Geometry check sheet. Reference: the model listing, model coordinates, mm. A direction names the side the tool comes from. Give positions to 0.01 mm unless a question says otherwise; leave off trailing zeros. Write each loop counter-clockwise with the first axis right and the second up, starting at its lowest first coordinate (ties: lowest second). Pieces come first, ordered by that corner, then holes. Notation, with made-up numbers: (18, -24.5) - (65, -24.5) arc R29 cw to (65, 11.5) - close; hole circle Ø6 at (26.25, 44). An arc over 180 degrees is marked (long way). Write item = value, one per line. Start each with the question number.
(1) Depth check by flat-ended pin: pin 1 Ø0.5 at (x, y) = (9, 18) entering from +Z; pin 2 Ø8 at (x, y) = (-2.5, 9.5) entering from -Z; pin 3 Ø0.5 at (x, z) = (-13.5, -5.5) entering from -Y; pin 4 Ø3.5 at (x, z) = (-12, 1) entering from +Y. Enter the tip coordinate at first touch or a pass-through.
(2) Thickness scan on L1, parallel to X at y = 14.5, z = 6; L2, parallel to X at y = 14.25, z = 21; L3, parallel to Z at x = -5.5, y = 11.75. Record the ranges inside material, lowest first.
(3) Section check A-A, the plane y = 19.75. Enter the section's corners in (x, z), plus the area to 3 significant figures.
(4) Access from +Z, -Z, +X, -X, +Y, -Y to the whole of each face (thin tool, end or side, straight path). Record for faces 1 (the flat face through (13, 21, 18)), 2 (the flat face through (12, 19, 23)), 3 (the flat face through (13.5, 18, -18)), 4 (the cylindrical face through (-0.037, 13.325, -19.232)).
(5) Draft check along X on faces 5 (the cylindrical face through (0.19, 0.45, -19.57)), 6 (the flat face through (-13.75, 21.5, -7.6)), 7 (the cylindrical face through (-0.163, 7.526, -19.232)). Enter one of: pulls with the +X half, pulls with the -X half, needs draft (parallel to the pull), parting line crosses it, or undercut.
```python
from build123d import *

# Parameters (mm, degrees)
BOSS_EXTRUDE1_DEPTH      = 17.5
CUT_EXTRUDE1_DEPTH       = 14
CUT_EXTRUDE2_DEPTH       = 54.247065647
SKETCH4_W                = 26
SKETCH4_H                = 8
CUT_EXTRUDE3_DEPTH       = 1
BOSS_EXTRUDE3_DEPTH      = 7.5
BOSS_EXTRUDE3_DEPTH_BACK = 1
SKETCH6_W                = 5.4
SKETCH6_H                = 36
FILLET2_R                = 2
FILLET5_R                = 1.5
SKETCH13_W               = 15.2
SKETCH13_H               = 28
BOSS_EXTRUDE7_DEPTH      = 4
SKETCH15_R               = 1
CUT_EXTRUDE8_DEPTH       = 6
CHAMFER5_SIZE            = 6
SKETCH16_W               = 11
SKETCH16_H               = 5.5
BOSS_EXTRUDE8_DEPTH      = 2
SKETCH17_W               = 11
SKETCH17_H               = 5.5
BOSS_EXTRUDE9_DEPTH      = 2
BOSS_EXTRUDE14_START     = -2
BOSS_EXTRUDE14_DEPTH     = 0.5
CHAMFER6_SIZE            = 0.5
BOSS_EXTRUDE15_DEPTH     = 0.5
CHAMFER7_SIZE            = 0.5
CUT_EXTRUDE9_REACH       = 59.483
BOSS_EXTRUDE16_DEPTH     = 1
FILLET7_R                = 1
SKETCH27_W               = 11
SKETCH27_H               = 2
BOSS_EXTRUDE17_DEPTH     = 0.75
SKETCH27_3_W             = 11
SKETCH27_3_H             = 2.5
CUT_EXTRUDE10_DEPTH      = 0.3
SKETCH29_W               = 11
SKETCH29_H               = 2
BOSS_EXTRUDE18_DEPTH     = 0.75
SKETCH29_4_W             = 11
SKETCH29_4_H             = 2.5
CUT_EXTRUDE11_DEPTH      = 0.3
FILLET8_R                = 1


# Some blends are built 0.0001 mm under size
with BuildPart() as part:
    # Sketch1 → Boss-Extrude1 (new body)
    with BuildSketch(Plane(origin=(0, 0, 0), x_dir=(1, 0, 0), z_dir=(0, 1, 0))):
        Polygon((-15, 20), (15, 20), (15, -20), (15, -30), (-15, -30), (-15, -20), align=None)
    extrude(amount=BOSS_EXTRUDE1_DEPTH)

    # Sketch2 → Cut-Extrude1 (cut)
    with BuildSketch(Plane(origin=(0, 17.5, 0), x_dir=(1, 0, 0), z_dir=(0, 1, 0))):
        Polygon((-13, 18), (13, 18), (13, -18), (13, -28), (-13, -28), (-13, -18), align=None)
    extrude(amount=-CUT_EXTRUDE1_DEPTH, mode=Mode.SUBTRACT)

    # Sketch3 → Cut-Extrude2 (cut, through all)
    with BuildSketch(Plane.XY.offset(-18)):
        with BuildLine():
            ThreePointArc((2.74956137, 10.425664385), (-0.1, 13.325664385), (-2.94956137, 10.425664385))
            ThreePointArc((-2.94956137, 10.425664385), (-0.1, 7.525664385), (2.74956137, 10.425664385))
        make_face()
    extrude(amount=-CUT_EXTRUDE2_DEPTH, mode=Mode.SUBTRACT)

    # Sketch4 → Cut-Extrude3 (cut)
    with BuildSketch(Plane(origin=(0, 3.5, 0), x_dir=(1, 0, 0), z_dir=(0, 1, 0))):
        with Locations((0, 14)):
            Rectangle(SKETCH4_W, SKETCH4_H)
    extrude(amount=-CUT_EXTRUDE3_DEPTH, mode=Mode.SUBTRACT)

    # Sketch6 → Boss-Extrude3 (add, two sides: drawn at the far end of the back side and taken through both)
    with BuildSketch(Plane(origin=(0, 3.5, 0), x_dir=(1, 0, 0), z_dir=(0, 1, 0)).offset(-BOSS_EXTRUDE3_DEPTH_BACK)):
        with Locations((-10.3, 0)):
            Rectangle(SKETCH6_W, SKETCH6_H)
        with Locations((10.3, 0)):
            Rectangle(SKETCH6_W, SKETCH6_H)
    extrude(amount=BOSS_EXTRUDE3_DEPTH + BOSS_EXTRUDE3_DEPTH_BACK)

    # Fillet2
    fillet2_edges = [part.edges().sort_by_distance(p)[0] for p in [
        (-7.6, 11, 0),
        (7.6, 11, 0),
    ]]
    fillet(fillet2_edges, radius=FILLET2_R)

    # Fillet5
    fillet5_edges = [part.edges().sort_by_distance(p)[0] for p in [
        (15, 8.75, 30),
        (-15, 8.75, 30),
        (-15, 8.75, -20),
        (15, 8.75, -20),
        (0, 0, 30),
        (-15, 0, 5),
        (0, 0, -20),
        (15, 0, 5),
    ]]
    fillet(fillet5_edges, radius=FILLET5_R)

    # Sketch13 → Boss-Extrude7 (add)
    with BuildSketch(Plane(origin=(0, 3.5, 0), x_dir=(1, 0, 0), z_dir=(0, 1, 0))):
        with Locations((0, -4)):
            Rectangle(SKETCH13_W, SKETCH13_H)
    extrude(amount=BOSS_EXTRUDE7_DEPTH)

    # Sketch15 → Cut-Extrude8 (cut)
    with BuildSketch(Plane(origin=(0, 7.5, 0), x_dir=(1, 0, 0), z_dir=(0, 1, 0))):
        with Locations(Location((0, -8.82, 0), (0, 0, 270))):
            Circle(SKETCH15_R)
    extrude(amount=-CUT_EXTRUDE8_DEPTH, mode=Mode.SUBTRACT)

    # Chamfer5
    # the kernel refuses this chamfer: 6 mm, written as the material it takes off along each edge
    with BuildSketch(Plane(origin=(-7.6, 7.5, -10), x_dir=(0, -0.9996219169112968, -0.02749587661058649), z_dir=(1, 0, 0))) as chamfer5_piece_1_section:
        Polygon((CHAMFER5_SIZE * 0.999621916911, -CHAMFER5_SIZE * 0.0274958766106), (-CHAMFER5_SIZE * 0.0274958766106, -CHAMFER5_SIZE * 0.999621916911), (0, 0), align=None)
    chamfer5_piece_1 = extrude(amount=15.2, mode=Mode.PRIVATE)
    chamfer5_piece_1 = split(chamfer5_piece_1, bisect_by=Plane(origin=(0, 2.5, -7.952380952), z_dir=(0, 1, 0)), keep=Keep.TOP, mode=Mode.PRIVATE)
    add(chamfer5_piece_1, mode=Mode.SUBTRACT)

    # Sketch16 → Boss-Extrude8 (add)
    with BuildSketch(Plane(origin=(-13, 0, 0), x_dir=(0, 0, -1), z_dir=(1, 0, 0))):
        Polygon((2, 17.5), (2, 14.5), (2, 12), (13, 12), (13, 14.5), (13, 17.5), align=None)
        with Locations((7.5, 20.25)):
            Rectangle(SKETCH16_W, SKETCH16_H)
    extrude(amount=BOSS_EXTRUDE8_DEPTH)

    # Sketch17 → Boss-Extrude9 (add)
    with BuildSketch(Plane.ZY.offset(-13)):
        with Locations((17.5, 20.25)):
            Rectangle(SKETCH17_W, SKETCH17_H)
        Polygon((12, 17.5), (12, 14.5), (12, 12), (23, 12), (23, 14.5), (23, 17.5), align=None)
    extrude(amount=BOSS_EXTRUDE9_DEPTH)

    # Sketch3<4> → Boss-Extrude14 (add)
    with BuildSketch(Plane.XY.offset(-18).offset(BOSS_EXTRUDE14_START)):
        Polygon((-4.129390667, 8.806636123), (-1.769028262, 6.446273719), (1.569028262, 6.446273719), (3.929390667, 8.806636123), (3.929390667, 12.144692648), (1.569028262, 14.505055052), (-1.769028262, 14.505055052), (-4.129390667, 12.144692648), align=None)
        with BuildLine():
            ThreePointArc((-2.94956137, 10.425664385), (-0.1, 7.525664385), (2.74956137, 10.425664385))
            ThreePointArc((2.74956137, 10.425664385), (-0.1, 13.325664385), (-2.94956137, 10.425664385))
        make_face(mode=Mode.SUBTRACT)
    extrude(amount=-BOSS_EXTRUDE14_DEPTH)

    # Chamfer6
    chamfer6_edges = [part.edges().sort_by_distance(p)[0] for p in [
        (2.749209465, 13.32487385, -20.5),
        (3.929390667, 10.475664385, -20.5),
        (2.749209465, 7.626454921, -20.5),
        (-0.1, 6.446273719, -20.5),
        (-2.949209465, 7.626454921, -20.5),
        (-4.129390667, 10.475664385, -20.5),
        (-2.949209465, 13.32487385, -20.5),
        (-0.1, 14.505055052, -20.5),
    ]]
    chamfer(chamfer6_edges, length=CHAMFER6_SIZE - 0.0001)  # a hair under: the kernel refuses the full size

    # Sketch23 → Boss-Extrude15 (add)
    with BuildSketch(Plane.XZ):
        Polygon((-12, 17), (-12, -17), (12, -17), (12, 17), (12, 27), (-12, 27), align=None)
    extrude(amount=BOSS_EXTRUDE15_DEPTH)

    # Chamfer7
    chamfer7_edges = [part.edges().sort_by_distance(p)[0] for p in [
        (12, -0.5, 5),
        (-12, -0.5, 5),
        (0, -0.5, -17),
        (0, -0.5, 27),
    ]]
    chamfer(chamfer7_edges, length=CHAMFER7_SIZE - 0.0001)  # a hair under: the kernel refuses the full size

    # Sketch24 → Cut-Extrude9 (cut, up to next)
    with BuildSketch(Plane.XY.offset(30), mode=Mode.PRIVATE) as cut_extrude9_sk1:
        with BuildLine():
            Line((-3, 17.5), (3, 17.5))
            ThreePointArc((3, 17.5), (0, 14.5), (-3, 17.5))
        make_face()
    cut_extrude9_tool1 = extrude(cut_extrude9_sk1.sketch, amount=-CUT_EXTRUDE9_REACH, mode=Mode.PRIVATE) & part.part
    add(cut_extrude9_tool1.solids().sort_by_distance((0, 16.22676, 30))[0], mode=Mode.SUBTRACT)

    # Sketch26 → Boss-Extrude16 (add)
    with BuildSketch(Plane(origin=(0, 17.5, 0), x_dir=(1, 0, 0), z_dir=(0, 1, 0))):
        Polygon((-13, 13), (-13, 18), (-14, 18), (-14, -19.115845085), (-14, -28.884154915), (-3, -28.884154915), (-3, -28), (-13, -28), (-13, 2), align=None)
        Polygon((3, -28), (13, -28), (13, 18), (14, 18), (14, -28.884154915), (3, -28.884154915), align=None)
    extrude(amount=BOSS_EXTRUDE16_DEPTH)

    # Fillet7
    fillet7_edges = [part.edges().sort_by_distance(p)[0] for p in [
        (-13, 15.25, -13),
        (-13, 15.25, -2),
        (-13, 12, -7.5),
        (13, 15.25, 12),
        (13, 12, 17.5),
        (13, 15.25, 23),
        (0, 3.5, 18),
    ]]
    fillet(fillet7_edges, radius=FILLET7_R - 0.0001)  # a hair under: the kernel refuses the full size

    # Sketch27 → Boss-Extrude17 (add)
    with BuildSketch(Plane.ZY.offset(13)):
        with Locations((-7.5, 22)):
            Rectangle(SKETCH27_W, SKETCH27_H)
    extrude(amount=BOSS_EXTRUDE17_DEPTH)

    # Sketch27<3> → Cut-Extrude10 (cut)
    with BuildSketch(Plane.ZY.offset(13)):
        with Locations((-7.5, 19.75)):
            Rectangle(SKETCH27_3_W, SKETCH27_3_H)
    extrude(amount=-CUT_EXTRUDE10_DEPTH, mode=Mode.SUBTRACT)

    # Sketch29 → Boss-Extrude18 (add)
    with BuildSketch(Plane(origin=(13, 0, 0), x_dir=(0, 0, -1), z_dir=(1, 0, 0))):
        with Locations((-17.5, 22)):
            Rectangle(SKETCH29_W, SKETCH29_H)
    extrude(amount=BOSS_EXTRUDE18_DEPTH)

    # Sketch29<4> → Cut-Extrude11 (cut)
    with BuildSketch(Plane(origin=(13, 0, 0), x_dir=(0, 0, -1), z_dir=(1, 0, 0))):
        with Locations((-17.5, 19.75)):
            Rectangle(SKETCH29_4_W, SKETCH29_4_H)
    extrude(amount=-CUT_EXTRUDE11_DEPTH, mode=Mode.SUBTRACT)

    # Fillet8
    fillet8_edges = [part.edges().sort_by_distance(p)[0] for p in [
        (-11, 23, -7.5),
        (11, 23, 17.5),
        (-13.75, 23, -7.5),
        (13.75, 23, 17.5),
    ]]
    fillet(fillet8_edges, radius=FILLET8_R)


solid = part.part
```
Model answer:
q1.pin_1 = 28.88
q1.pin_2 = -20.5
q1.pin_3 = 0
q1.pin_4 = 18.5
q2.L1 = -15 to -13, 13 to 15
q2.L2 = -15 to -13, 11 to 15
q2.L3 = -20 to -18, 28 to 30
q3.outline = (-12.7, -13) - (-11, -13) - (-11, -2) - (-12.7, -2) - close; (11, 12) - (12.7, 12) - (12.7, 23) - (11, 23) - close
q3.area = 37.4 mm²
q4.face_1 = +Z, -Z, +X
q4.face_2 = +Y
q4.face_3 = -Z, +X, -X, +Y
q4.face_4 = -Z
q5.face_5 = needs draft
q5.face_6 = pulls with the -X half
q5.face_7 = undercut
